Can you work these out from the model? Positions are in its coordinate system, mm. Face numbers are marked on the shaded views. A direction names the side the tool comes from. Coordinates: 2 decimals unless noted, no trailing zeros. Order: outer loops, then holes, each group sorted by start corner. A loop starts at its lowest first (then second) coordinate and runs counter-clockwise, first axis right, second up. Notation, with made-up numbers: M 39.25,74 L 74.25,74 A12 cw 74.25,79 Z; hole C 72.5,65 d2. An arc over 180 degrees is marked long. Answer as a JSON object with one key per item and string values.
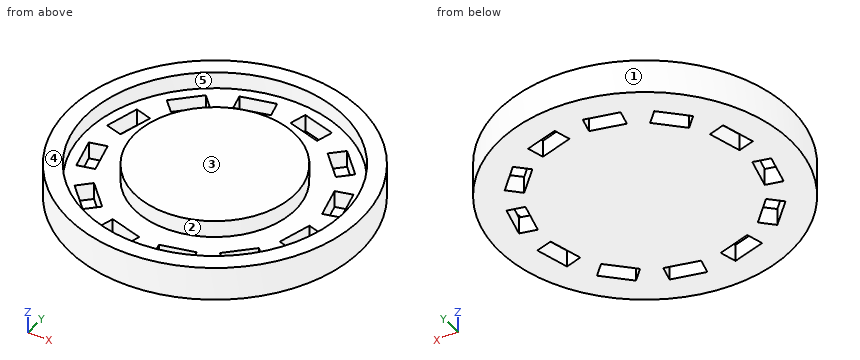
from build123d import *

# Parameters (mm, degrees)
SKETCH004_R        = 8.65
PAD003_DEPTH       = 2
SKETCH005_R        = 7.65
POCKET_DEPTH       = 1
SKETCH006_W        = 1
SKETCH006_H        = 2
POCKET001_DEPTH    = 50.09601
POLARPATTERN_COUNT = 12
SKETCH007_R        = 4.75
PAD004_DEPTH       = 1


with BuildPart() as part:
    # Sketch004 → Pad003 (new body)
    with BuildSketch(Plane(origin=(0, 0, 12.1), x_dir=(0, 1, 0), z_dir=(0, 0, 1))):
        Circle(SKETCH004_R)
    extrude(amount=PAD003_DEPTH)

    # Sketch005 (on Face3 of Pad003) → Pocket (cut)
    with BuildSketch(Plane.XY.offset(14.1)):
        Circle(SKETCH005_R)
    extrude(amount=-POCKET_DEPTH, mode=Mode.SUBTRACT)

    # Sketch006 (on Face5 of Pocket) → Pocket001 (cut, through all)
    with BuildSketch(Plane(origin=(0, 0, 13.1), x_dir=(0.707107, 0.707107, 0), z_dir=(0, 0, 1))):
        with Locations((-6.5, 0)):
            Rectangle(SKETCH006_W, SKETCH006_H)
    pocket001 = extrude(amount=-POCKET001_DEPTH, mode=Mode.SUBTRACT)

    # PolarPattern: Pocket001 ×12 about axis
    polarpattern_axis = Axis((0, 0, 13.1), (0, 0, 1))
    for i in range(1, POLARPATTERN_COUNT):
        add(pocket001.rotate(polarpattern_axis, i * 360 / POLARPATTERN_COUNT), mode=Mode.SUBTRACT)

    # Sketch007 (on Face53 of PolarPattern) → Pad004 (join)
    with BuildSketch(Plane(origin=(0, 0, 13.1), x_dir=(0, 1, 0), z_dir=(0, 0, 1))):
        Circle(SKETCH007_R)
    extrude(amount=PAD004_DEPTH)


solid = part.part
Item 1: If we mould it in two halves opening along Y, with no side actions, what happens to the marked faces 1, 2 and 3? For each: pulls with the +Y half, pulls with the -Y half, needs draft (parallel to the pull), parting line crosses it, or undercut.
Answers follow:
{"face 1": "parting line crosses it", "face 2": "undercut", "face 3": "needs draft"}
Item 2: I want a section at B-B, the plane y = 0. Write out the boundary of the cut face in (x, z).
Answers follow:
{"outline": "M -8.65,12.1 L 8.65,12.1 L 8.65,14.1 L 7.65,14.1 L 7.65,13.1 L 4.75,13.1 L 4.75,14.1 L -4.75,14.1 L -4.75,13.1 L -7.65,13.1 L -7.65,14.1 L -8.65,14.1 Z"}
Item 3: Please list where these lines run through material, in increasing order: line 1 (Y direction, x = 0, z = 13.9); line 2 (X direction, y = -5.5, z = 12.7); line 3 (Y direction, x = -2.25, z = 13.45).
Answers follow:
{"line 1": "y = -8.65 to -7.65, -4.75 to 4.75, 7.65 to 8.65", "line 2": "x = -6.68 to -4.4, -4.09 to 4.09, 4.4 to 6.68", "line 3": "y = -8.35 to -7.31, -4.18 to 4.18, 7.31 to 8.35"}
Item 4: I want a section at A-A, the plane y = 5.25. Write out the boundary of the cut face in (x, z).
Answers follow:
{"outline": "M -6.87,12.1 L -4.65,12.1 L -4.65,13.1 L -5.56,13.1 L -5.56,14.1 L -6.87,14.1 Z; M -3.84,12.1 L 3.84,12.1 L 3.84,13.1 L -3.84,13.1 Z; M 4.65,12.1 L 6.87,12.1 L 6.87,14.1 L 5.56,14.1 L 5.56,13.1 L 4.65,13.1 Z"}
Item 5: I want a section at D-D, the plane z = 12.3. Give the number of separate pieces and of enclosed holes in the cut face, plus the area to 3 significant figures.
Answers follow:
{"separate pieces": "1", "enclosed holes": "12", "area": "211 mm^2"}
Item 6: Which directions (+Z, -Z, +X, -X, +Y, -Y) give clear straight access to the entire face, cutting with the end or side of a thin tool? Please do the marked faces 4 and 5.
Answers follow:
{"face 4": "+Z, +X, -X, +Y, -Y", "face 5": "+Z"}
